```python
from build123d import *

# Parameters (mm, degrees)
SKETCH_1_W          = 20
SKETCH_1_H          = 21.4
EXTRUDE_1_DEPTH     = 5
SKETCH_4_R          = 0.85
CUT_EXTRUDE_1_DEPTH = 4
SKETCH_5_R          = 0.85
CUT_EXTRUDE_2_DEPTH = 4
SKETCH_6_W          = 21.4
SKETCH_6_H          = 5
EXTRUDE_2_DEPTH     = 2.5
SKETCH_7_R          = 2.6
CUT_EXTRUDE_3_DEPTH = 2.6


with BuildPart() as part:
    # 草图1 → 凸台-拉伸1 (new body)
    with BuildSketch(Plane(origin=(0, 0, 0), x_dir=(1, 0, 0), z_dir=(0, 1, 0))):
        with Locations((-10, -10.7)):
            Rectangle(SKETCH_1_W, SKETCH_1_H)
    extrude(amount=EXTRUDE_1_DEPTH)

    # 草图4 → 切除-拉伸1 (cut)
    with BuildSketch(Plane.ZY.offset(20)):
        with Locations((16.4, 2.5)):
            Circle(SKETCH_4_R)
        with Locations((5, 2.5)):
            Circle(SKETCH_4_R)
    extrude(amount=-CUT_EXTRUDE_1_DEPTH, mode=Mode.SUBTRACT)

    # 草图5 → 切除-拉伸2 (cut)
    with BuildSketch(Plane(origin=(0, 0, 0), x_dir=(-1, 0, 0), z_dir=(0, 0, -1))):
        with Locations((15, 2.5)):
            Circle(SKETCH_5_R)
        with Locations((5, 2.5)):
            Circle(SKETCH_5_R)
    extrude(amount=-CUT_EXTRUDE_2_DEPTH, mode=Mode.SUBTRACT)

    # 草图6 → 凸台-拉伸2 (add)
    with BuildSketch(Plane(origin=(0, 0, 0), x_dir=(0, 0, -1), z_dir=(1, 0, 0))):
        with Locations((-10.7, 2.5)):
            Rectangle(SKETCH_6_W, SKETCH_6_H)
    extrude(amount=EXTRUDE_2_DEPTH)

    # 草图7 → 切除-拉伸3 (cut)
    with BuildSketch(Plane(origin=(0, 5, 0), x_dir=(1, 0, 0), z_dir=(0, 1, 0))):
        with Locations(Location((-6, -13.9, 0), (0, 0, 270))):
            Circle(SKETCH_7_R)
    extrude(amount=-CUT_EXTRUDE_3_DEPTH, mode=Mode.SUBTRACT)


solid = part.part
```
CAD build for the part. Positions are in the model's coordinates, mm. A direction names the side the tool comes from. Coordinates: 2 decimals unless noted, no trailing zeros. Order: outer loops, then holes, each group sorted by start corner. A loop starts at its lowest first (then second) coordinate and runs counter-clockwise, first axis right, second up.
(1) Mould opens along X. For faces 5 (the face through (-9, 5, 11)), 6 (the face through (-15, 3, 4)), 7 (the face through (-16, 3, 16)), 8 (the face through (-6, 2.4, 14)) say: released by +X, released by -X, zero draft, split by the parting line, or undercut.
Solution:
face 5: zero draft
face 6: undercut
face 7: released by -X
face 8: undercut
(2) Saw through at B-B, the plane z = 3.5. Write the cut outline in (x, y).
Solution:
outline: (-20, 0) - (2.5, 0) - (2.5, 5) - (-20, 5) - close; hole circle Ø1.7 at (-15, 2.5); hole circle Ø1.7 at (-5, 2.5)
(3) Which spindle directions (+Z, -Z, +X, -X, +Y, -Y) get a long thin tool onto all of the face, cutting with end or side? Do faces 1 (the face through (-9, 2, 21.4)), 2 (the face through (-5.22, 3.72, 16.38)), 3 (the face through (-5, 3, 4)), 4 (the face through (-18.03, 1.67, 4.82)). Say none if no direction does.
Solution:
face 1: +Z, +X, -X, +Y, -Y
face 2: +Y
face 3: -Z
face 4: -X
(4) Saw through at A-A, the plane y = 4.7. Write the cut outline in (x, z), and give its area (3 significant figures).
Solution:
outline: (-20, 0) - (2.5, 0) - (2.5, 21.4) - (-20, 21.4) - close; hole circle Ø5.2 at (-6, 13.9)
area: 460 mm2
(5) Drill centre lines: L1, parallel to Y at x = -5, z = 2; L2, parallel to Y at x = -7.25, z = 12.25; L3, parallel to X at y = 4.2, z = 13.9. Where is each one in solid material? Low to high.
Solution:
L1: y = 0 to 1.65, 3.35 to 5
L2: y = 0 to 2.4
L3: x = -20 to -8.6, -3.4 to 2.5
(6) Saw through at C-C, the plane z = 13.9. Write the cut outline in (x, y).
Solution:
outline: (-20, 0) - (2.5, 0) - (2.5, 5) - (-3.4, 5) - (-3.4, 2.4) - (-8.6, 2.4) - (-8.6, 5) - (-20, 5) - close
(7) Saw through at D-D, the plane x = -15. Write the cut outline in (y, z), and give its area (3 significant figures).
Solution:
outline: (0, 0) - (1.65, 0) - (1.65, 4) - (3.35, 4) - (3.35, 0) - (5, 0) - (5, 21.4) - (0, 21.4) - close
area: 100 mm2
(8) Pin check, flat tips, straight feed: pin 1 Ø2 at (x, y) = (-5, 2.5) entering from -Z; pin 2 Ø0.8 at (x, y) = (-15, 2.5) entering from -Z; pin 3 Ø4 at (x, z) = (-6, 13.9) entering from +Y. Stop position of each tip, or through.
Solution:
pin 1: stops at z = 0
pin 2: stops at z = 4
pin 3: stops at y = 2.4
